Design review of the part built by this model. Coordinates are the model's own, in mm. Face numbers are marked on the shaded views. A direction names the side the tool comes from. Round coordinates to 2 decimals unless told otherwise and drop trailing zeros. Write each loop counter-clockwise with the first axis right and the second up, starting at its lowest first coordinate (ties: lowest second). Pieces come first, ordered by that corner, then holes. Notation, with made-up numbers: M -9,82 L -1,82 A13 ccw -1,100 Z; hole C 2.25,30.25 d7. An arc over 180 degrees is marked long. One line per question, with ' | ' between items. Start each with the question number.
Item 1: Draft analysis for pull direction Y (two halves, no side actions). For the marked faces 1, 2 and 3, state which applies: released by +Y, released by -Y, zero draft, split by the parting line, or undercut.
Item 2: Add section C-C, the plane z = -8.25. State the section outline as (x, y) points, and give its area (3 significant figures).
Item 3: Add section B-B, the plane y = -0.5. State the section outline as (x, z) points, and give its area (3 significant figures).
Item 4: Insertion check: pin 1 Ø1.5 at (x, z) = (4, -2.5) entering from -Y; pin 2 Ø6 at (x, z) = (3.5, -6.5) entering from +Y. Each pin has a flat end and moves straight along its axis. Give the tip position at first contact, or say it passes through.
Item 5: For L1, parallel to Y at x = -1.55, z = 0; L2, parallel to Y at x = 3.65, z = 0; L3, parallel to X at y = 7, z = 4.5, list the stretches that pass through material, from the lowest coordinate up.
Item 6: Add section D-D, the plane x = -0.5. State the section outline as (y, z) points.
Item 7: Add section A-A, the plane z = 0. State the section outline as (x, y) points.
Item 8: Machinability: for the marked faces 4, 5, 6, 7 and 8, which of the approach directions +Z, -Z, +X, -X, +Y, -Y give a long, thin tool a straight path to every point of the face, cutting with its end or side? Answer none if there is none.
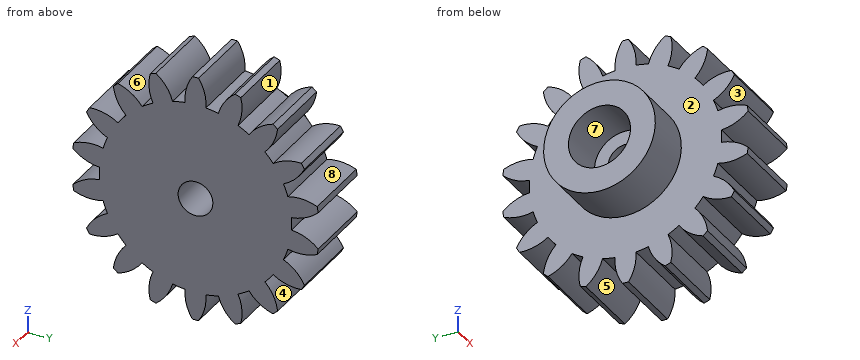
```python
from build123d import *

# Parameters (mm, degrees)
BASPROSKE_W         = 6
BASPROSKE_H         = 10
TOOTHCUT_DEPTH      = 16.362291496
TEETHCUTS_COUNT     = 18
TEETHCUTS_ANGLE     = 340
BORSKE_R            = 0.5
BORE_DEPTH          = 50.0000508
SKETCH3_R           = 2.3
BOSS_EXTRUDE3_DEPTH = 6
SKETCH1_R           = 4.5
BOSS_EXTRUDE4_DEPTH = 4
SKETCH4_R           = 2.5
CUT_EXTRUDE1_DEPTH  = 4
SKETCH5_R           = 1.4
CUT_EXTRUDE2_DEPTH  = 6


with BuildPart() as part:
    # BasProSke → Base-Revolve (revolve)
    with BuildSketch(Plane(origin=(0, 0, 0), x_dir=(1, 0, 0), z_dir=(0, 1, 0)), mode=Mode.PRIVATE) as base_revolve_sk:
        with Locations((3, 5)):
            Rectangle(BASPROSKE_W, BASPROSKE_H)
    revolve(base_revolve_sk.sketch.rotate(Axis((-10, 0, 0), (1, 0, 0)), 180), axis=Axis((-10, 0, 0), (1, 0, 0)))

    # TooCutSke → ToothCut (cut, through all)
    with BuildSketch(Plane(origin=(0, 0, 0), x_dir=(0, 0, -1), z_dir=(1, 0, 0))):
        with BuildLine():
            ThreePointArc((0.510641536, 7.732156635), (0, 7.749), (-0.510641536, 7.732156635))
            ThreePointArc((-0.510641536, 7.732156635), (-0.82619259, 8.907320741), (-1.515208602, 9.910236529))
            ThreePointArc((-1.515208602, 9.910236529), (0, 10.0254), (1.515208602, 9.910236529))
            ThreePointArc((1.515208602, 9.910236529), (0.82619259, 8.907320741), (0.510641536, 7.732156635))
        make_face()
    toothcut = extrude(amount=TOOTHCUT_DEPTH, mode=Mode.SUBTRACT)

    # TeethCuts: ToothCut ×18 about axis
    teethcuts_axis = Axis((-10, 0, 0), (1, 0, 0))
    for i in range(1, TEETHCUTS_COUNT):
        add(toothcut.rotate(teethcuts_axis, i * TEETHCUTS_ANGLE / (TEETHCUTS_COUNT - 1)), mode=Mode.SUBTRACT)

    # BorSke → Bore (cut, symmetric)
    with BuildSketch(Plane(origin=(0, 0, 0), x_dir=(0, 0, -1), z_dir=(1, 0, 0))):
        with Locations(Location((0, 0, 0), (0, 0, 180))):
            Circle(BORSKE_R)
    extrude(amount=BORE_DEPTH, both=True, mode=Mode.SUBTRACT)

    # Sketch3 → Boss-Extrude3 (add)
    with BuildSketch(Plane(origin=(6, 0, 0), x_dir=(0, 0, -1), z_dir=(1, 0, 0))):
        Circle(SKETCH3_R)
    extrude(amount=-BOSS_EXTRUDE3_DEPTH)

    # Sketch1 → Boss-Extrude4 (add)
    with BuildSketch(Plane.ZY):
        with Locations(Location((0, 0, 0), (0, 0, 180))):
            Circle(SKETCH1_R)
    extrude(amount=BOSS_EXTRUDE4_DEPTH)

    # Sketch4 → Cut-Extrude1 (cut)
    with BuildSketch(Plane.ZY.offset(4)):
        Circle(SKETCH4_R)
    extrude(amount=-CUT_EXTRUDE1_DEPTH, mode=Mode.SUBTRACT)

    # Sketch5 → Cut-Extrude2 (cut)
    with BuildSketch(Plane(origin=(6, 0, 0), x_dir=(0, 0, -1), z_dir=(1, 0, 0))):
        Circle(SKETCH5_R)
    extrude(amount=-CUT_EXTRUDE2_DEPTH, mode=Mode.SUBTRACT)


solid = part.part
```
Computed values:
1) face 1: undercut | face 2: zero draft | face 3: released by -Y
2) outline: M 0,-3.75 L 6,-3.75 L 6,-2.13 L 0,-2.13 Z; M 0,-0.84 L 6,-0.84 L 6,0.84 L 0,0.84 Z; M 0,2.13 L 6,2.13 L 6,3.75 L 0,3.75 Z | area: 29.5 mm^2
3) outline: M -4,-4.47 L 0,-4.47 L 0,-9.55 L 6,-9.55 L 6,-1.31 L 0,-1.31 L 0,-2.45 L -4,-2.45 Z; M -4,2.45 L 0,2.45 L 0,1.31 L 6,1.31 L 6,9.55 L 0,9.55 L 0,4.47 L -4,4.47 Z | area: 115 mm^2
4) pin 1: stops at y = -9.85 | pin 2: stops at y = 8.78
5) L1: y = -4.5 to -2.5, 2.5 to 4.5 | L2: y = -7.75 to -1.4, 1.4 to 7.75 | L3: x = 0 to 6
6) outline: C 0,0 d9; hole C 0,0 d5
7) outline: M -4,-4.5 L 0,-4.5 L 0,-7.75 L 6,-7.75 L 6,-1.4 L 0,-1.4 L 0,-2.5 L -4,-2.5 Z; M -4,2.5 L 0,2.5 L 0,1.4 L 6,1.4 L 6,7.75 L 0,7.75 L 0,4.5 L -4,4.5 Z
8) face 4: +X, -X, +Y | face 5: -Z, +X, -X | face 6: +Z, +X, -X | face 7: -X | face 8: +X, -X
